Answer from the drawing. Dimensions are ordinates in mm from the lowest x, y and z of the part. A direction names the side the tool comes from. Coordinates: 2 decimals unless noted, no trailing zeros. Write each loop counter-clockwise with the first axis right and the second up, starting at its lowest first coordinate (ties: lowest second). Pieces come first, ordered by that corner, then holes. Notation, with made-up numbers: (43.25, 18.25) - (84.25, 18.25) arc R20 cw to (84.25, 47.25) - close; hole circle Ø7 at (35, 76). An arc over 180 degrees is marked (long way). Use a Markdown table: item, result.
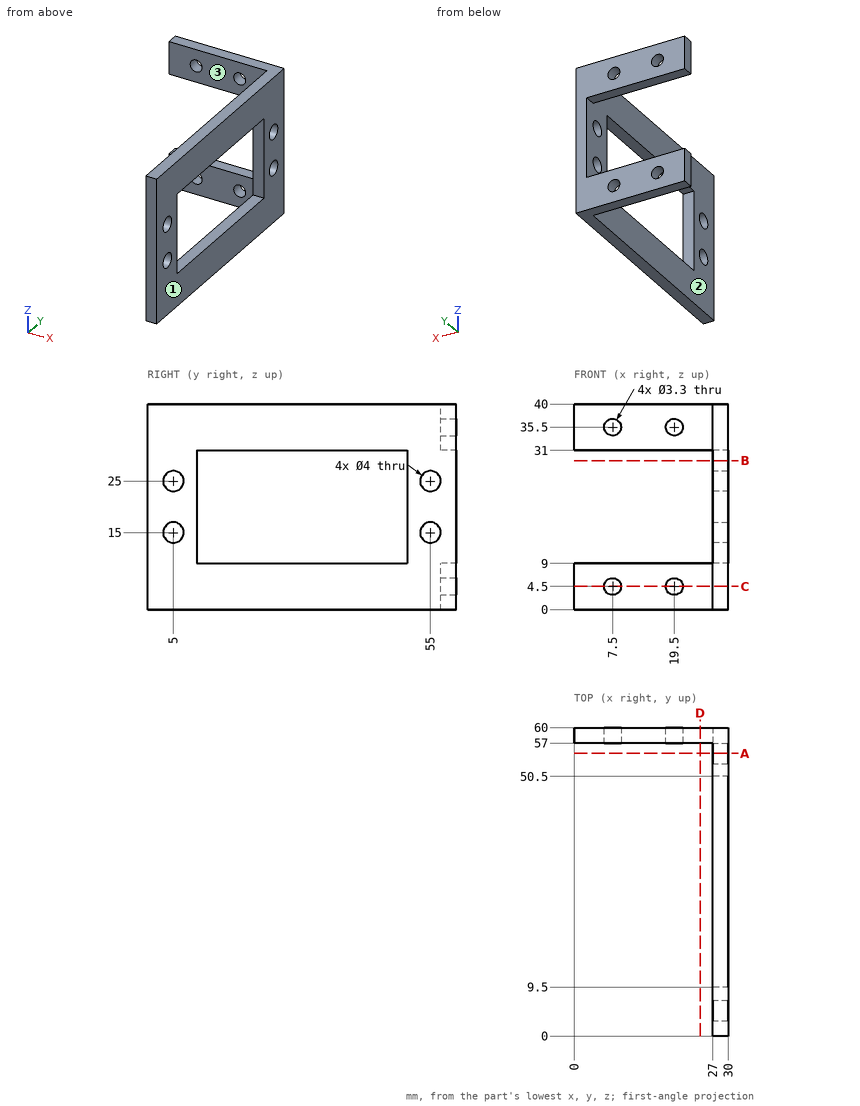
(1) Each of these flat-tipped pins is pushed along its axis until it touches: P1, Ø4.5, axis at x = 15.5, z = 5.5, coming from the -Y side; P2, Ø5, axis at y = 5, z = 25, coming from the -X side. Where does it stop, or does it pass through?
Report:
| item | result |
|---|---|
| P1 | stops at y = 57 |
| P2 | stops at x = 27 |
(2) For the marked faces 1, 2 and 3, determine the directions among +Z, -Z, +X, -X, +Y, -Y from which every point of the face is accessible in a straight line to the end or side of a thin tool.
Report:
| item | result |
|---|---|
| face 1 | +Z, -Z, +X, +Y, -Y |
| face 2 | -X, -Y |
| face 3 | +Z, -Z, -X, -Y |
(3) A cutting plane is placed at C-C, the plane z = 4.5. Write down the section's boundary in (x, y), and give its area (3 significant figures).
Report:
| item | result |
|---|---|
| outline | (0, 57) - (5.85, 57) - (5.85, 60) - (0, 60) - close; (9.15, 57) - (17.85, 57) - (17.85, 60) - (9.15, 60) - close; (21.15, 57) - (27, 57) - (27, 0) - (30, 0) - (30, 60) - (21.15, 60) - close |
| area | 241 mm² |
(4) A cutting plane is placed at B-B, the plane z = 29. Write down the section's boundary in (x, y).
Report:
| item | result |
|---|---|
| outline | (27, 0) - (30, 0) - (30, 9.5) - (27, 9.5) - close; (27, 50.5) - (30, 50.5) - (30, 60) - (27, 60) - close |
(5) Straight lines are drawn through the part: L1, parallel to X at y = 57.8, z = 4.5; L2, parallel to Y at x = 28.15, z = 15; L3, parallel to Y at x = 28, z = 27.5. For each, find the intervals that lie inside material, in ascending order.
Report:
| item | result |
|---|---|
| L1 | x = 0 to 5.85, 9.15 to 17.85, 21.15 to 30 |
| L2 | y = 0 to 3, 7 to 9.5, 50.5 to 53, 57 to 60 |
| L3 | y = 0 to 9.5, 50.5 to 60 |
(6) A cutting plane is placed at D-D, the plane x = 24.5. Write down the section's boundary in (y, z), and give its area (3 significant figures).
Report:
| item | result |
|---|---|
| outline | (57, 0) - (60, 0) - (60, 9) - (57, 9) - close; (57, 31) - (60, 31) - (60, 40) - (57, 40) - close |
| area | 54.0 mm² |
(7) A cutting plane is placed at A-A, the plane y = 55. Write down the section's boundary in (x, z).
Report:
| item | result |
|---|---|
| outline | (27, 0) - (30, 0) - (30, 13) - (27, 13) - close; (27, 17) - (30, 17) - (30, 23) - (27, 23) - close; (27, 27) - (30, 27) - (30, 40) - (27, 40) - close |
